Autodesk Inventor part; units mm, degrees
ref_plane "YZ Plane" through (0, 0, 0) normal (1, 0, 0) x (0, 1, 0)
ref_plane "XZ Plane" through (0, 0, 0) normal (0, 1, 0) x (-1, 0, 0)
ref_plane "XY Plane" through (0, 0, 0) normal (0, 0, 1) x (1, 0, 0)
sketch "Skizze4" plane through (0, 0, 0) normal (0, 0, 1) x (1, 0, 0)
  circle A0 centre (0, 25) radius 4 construction
  circle A1 centre (0, -25) radius 4 construction
  circle A2 centre (0, 0) radius 3 construction
  line L0 (-11.0333, -36.517) -> (-22.869, -57.017) construction
  line L1 (12.638, -36.517) -> (-11.0333, -36.517) construction
  line L2 (24.4737, -57.017) -> (12.638, -36.517) construction
  line L3 (12.638, -77.517) -> (24.4737, -57.017) construction
  circle A3 centre (0.8023, -57.017) radius 18 construction
  line L4 (12.638, -36.517) -> (-11.0333, -36.517) construction
  line L5 (-11.0333, -36.517) -> (-22.869, -57.017) construction
  line L6 (-22.869, -57.017) -> (-11.0334, -77.517) construction
  line L7 (-11.0334, -77.517) -> (12.638, -77.517) construction
  line L8 (12.638, -77.517) -> (24.4737, -57.017) construction
  line L9 (24.4737, -57.017) -> (12.638, -36.517) construction
  circle A4 centre (0, 25) radius 4.3
  circle A5 centre (0, -25) radius 4.3
  circle A6 centre (0, 0) radius 4
  circle A7 centre (0, 25) radius 8 construction
  circle A8 centre (0, -25) radius 8
  circle A9 centre (0, -25) radius 8.3
  circle A10 centre (0, 25) radius 8.3
  line L10 (-13, 35) -> (13, 35)
  line L11 (13, 35) -> (13, -35)
  line L12 (13, -35) -> (-13, -35)
  line L13 (-13, -35) -> (-13, 35)
  line L14 (-13, 35) -> (13, -35) construction
  line L15 (13, 35) -> (-13, -35) construction
  line L16 (-13, -35) -> (-25.7115, -57.017)
  line L17 (-13, -35) -> (12.423, -35) construction
  line L18 (-25.7115, -57.017) -> (-25.7115, -71.017)
  line L19 (-25.7115, -71.017) -> (-29.7115, -71.017)
  line L20 (-29.7115, -71.017) -> (-29.7115, -57.017)
  line L21 (-29.7115, -57.017) -> (-13, -28.0718)
  line L22 (13, -35) -> (25.7115, -57.017)
  line L23 (13, -35) -> (38.423, -35) construction
  line L24 (25.7115, -57.017) -> (25.7115, -71.017)
  line L25 (25.7115, -71.017) -> (29.7115, -71.017)
  line L26 (29.7115, -71.017) -> (29.7115, -57.017)
  line L27 (29.7115, -57.017) -> (13, -28.0718)
  point P0 (0, 0)
  dimension "d22" = 0.3
  dimension "d23" = 0.3
  dimension "d24" = 1
  dimension "d25" = 0.3
  dimension "d26" = 0.3
  dimension "d27" = 26
  dimension "d28" = 70
  dimension "d29" = 120
  dimension "d30" = 14
  dimension "d31" = 4
  dimension "d32" = 90
  dimension "d33" = 60
  dimension "d34" = 4
  dimension "d35" = 90
  dimension "d36" = 150
  dimension "d46" = 12.7115
  dimension "d47" = 0
extrude "Extrusion4" add sketch "Skizze4" along normal up to surface (5.1 mm away) contours L10 L11 L12 L13 | L13 L16 L18 L19 L20 L21 | L27 L26 L25 L24 L22 L11
sketch "Skizze5" plane through (-13, -35, 5.1) normal (0, 0, 1) x (1, 0, 0)
  circle A0 centre (13, 60) radius 4 construction
  circle A1 centre (13, 10) radius 4 construction
  circle A2 centre (13, 60) radius 8.3
  circle A3 centre (13, 10) radius 8.3
  circle A4 centre (13, 35) radius 4
  line L0 (26, 0) -> (0, 0)
  line L1 (38.7115, -22.017) -> (26, 0)
  line L2 (38.7115, -36.017) -> (38.7115, -22.017)
  line L3 (42.7115, -36.017) -> (38.7115, -36.017)
  line L4 (42.7115, -22.017) -> (42.7115, -36.017)
  line L5 (26, 6.9282) -> (42.7115, -22.017)
  line L6 (26, 70) -> (26, 6.9282)
  line L7 (0, 70) -> (26, 70)
  line L8 (0, 6.9282) -> (0, 70)
  line L9 (-16.7115, -22.017) -> (0, 6.9282)
  line L10 (-16.7115, -36.017) -> (-16.7115, -22.017)
  line L11 (-12.7115, -36.017) -> (-16.7115, -36.017)
  line L12 (-12.7115, -22.017) -> (-12.7115, -36.017)
  line L13 (0, 0) -> (-12.7115, -22.017)
  circle A5 centre (13, 60) radius 4.4
  circle A6 centre (13, 10) radius 4.4
  point P0 (13, 35)
  dimension "d39" = 0.4
  dimension "d40" = 0.4
extrude "Extrusion5" add sketch "Skizze5" along normal blind 1 contours A2 | A3 | L0 L13 L12 L11 L10 L9 L8 L7 L6 L5 L4 L3 L2 L1
shell "Wandung1" thickness 2 removed faces 1 at (-11.3529, 9.9806, 0)
sketch "Skizze6" plane through (0, 0, 0) normal (0, 0, -1) x (-1, 0, 0)
  circle A0 centre (0, -25) radius 4.4
  circle A1 centre (0, -25) radius 8.3
  arc A2 (-6.4877, 33) -> (6.4877, 33) centre (0, 25) ccw
  circle A3 centre (0, 25) radius 4.4
  circle A4 centre (0, 25) radius 8.3
  arc A5 (6.4877, -33) -> (-6.4877, -33) centre (0, -25) ccw
  circle A6 centre (0, -25) radius 10.3
  circle A7 centre (0, 25) radius 10.3
  point P0 (0, 0)
extrude "Extrusion6" add sketch "Skizze6" along normal blind 2 contours A7 A2 | A6 A5
sketch "Skizze7" plane through (0, 0, 0) normal (0, 0, -1) x (-1, 0, 0)
  circle A0 centre (0, 0) radius 4
  circle A1 centre (0, 0) radius 6
  point P0 (0, 0)
extrude "Extrusion7" add sketch "Skizze7" along normal blind 3
properties part number "28_Z_Stage"
Input: part model. Units: mm. Frame: model coordinates. A direction names the side the tool comes from. Coordinates: 2 decimals unless noted, no trailing zeros. Write each loop counter-clockwise with the first axis right and the second up, starting at its lowest first coordinate (ties: lowest second). Pieces come first, ordered by that corner, then holes. Notation, with made-up numbers: M 28,-18.75 L 62,-18.75 A16 ccw 62,-1.75 Z; hole C -4.75,7 d1. An arc over 180 degrees is marked long. Use one line per item in the form item = value.
Q1. First-contact query: pin 1 (3 mm diameter, centred on y = -7, z = 0, fed in from +X); pin 2 (4.5 mm diameter, centred on y = -9.5, z = 2, fed in from -X); pin 3 (1.5 mm diameter, centred on x = 1, z = -0.5, fed in from +Y). Flat tips, straight axial feed; report the tip coordinate or a pass-through.
Answer below:
pin_1 = 13
pin_2 = -13
pin_3 = 35.3
Q2. Section D-D (y = -25). Return loops of the section in (x, z), plus the area to 3 significant figures.
Answer below:
outline = M -13,0 L -11,0 L -11,4.1 L -10.3,4.1 L -10.3,-2 L -8.3,-2 L -8.3,5.1 L -4.4,5.1 L -4.4,6.1 L -13,6.1 Z; M 4.4,5.1 L 8.3,5.1 L 8.3,-2 L 10.3,-2 L 10.3,4.1 L 11,4.1 L 11,0 L 13,0 L 13,6.1 L 4.4,6.1 Z
area = 67.4 mm²
Q3. Material intervals for probe 1 along Y at (x, z) = (0, 3.2); probe 2 along Y at (x, z) = (0, 5.4); probe 3 along X at (y, z) = (25, 2), sorted ascending. Write a range as from..to.
Answer below:
probe_1 = -35..-33.3, -16.7..-14.7, -6..-4, 4..6, 14.7..16.7, 33.3..35
probe_2 = -35..-29.4, -20.6..-4, 4..20.6, 29.4..35
probe_3 = -13..-11, -10.3..-8.3, 8.3..10.3, 11..13
Q4. Set-up query: faces 1 (the face through (-19.267, -45.854, 3.007)), 2 (the face through (-0.1, -35.3, -1)), 3 (the face through (12.25, -30.77, 2.08)), 4 (the face through (7, 30, -2)), 5 (the face through (0.1, 35.3, -1)). Return all of +Z, -Z, +X, -X, +Y, -Y with unobstructed straight access to the full face (end or side cutting, diameter ignored); none if empty.
Answer below:
face_1 = +Z, -Z, -Y
face_2 = -Z, -Y
face_3 = -Z
face_4 = -Z, +X, -X, +Y
face_5 = -Z, +Y
Q5. Section B-B (y = 0). Return loops of the section in (x, z), plus the area to 3 significant figures.
Answer below:
outline = M -13,0 L -11,0 L -11,4.1 L -6,4.1 L -6,-3 L -4,-3 L -4,6.1 L -13,6.1 Z; M 4,-3 L 6,-3 L 6,4.1 L 11,4.1 L 11,0 L 13,0 L 13,6.1 L 4,6.1 Z
area = 80.8 mm²
Q6. Section C-C (x = 0). Count the separate pieces of the cut face and the enclosed holes in it, plus the area to 3 significant figures.
Answer below:
separate_pieces = 4
enclosed_holes = 0
area = 148 mm²
Q7. Section A-A (z = 2.5). Return loops of the section in (x, y).
Answer below:
outline = M -29.71,-71.02 L -25.71,-71.02 L -25.71,-57.02 L -13,-35 L 13,-35 L 25.71,-57.02 L 25.71,-71.02 L 29.71,-71.02 L 29.71,-57.02 L 13,-28.07 L 13,35 L -13,35 L -13,-28.07 L -29.71,-57.02 Z; C 0,0 d12; hole M -13.54,-33 L -6.49,-33 A10.3 cw long 6.49,-33 L 13.54,-33 L 11,-28.61 L 11,33 L 6.49,33 A10.3 cw long -6.49,33 L -11,33 L -11,-28.61 Z; hole C 0,-25 d16.6; hole C 0,25 d16.6; hole C 0,0 d8
